Geometry: final body of the model. Coordinates: model frame, mm. A direction names the side the tool comes from. Give positions to 0.01 mm unless a question says otherwise; leave off trailing zeros. Write each loop counter-clockwise with the first axis right and the second up, starting at its lowest first coordinate (ties: lowest second). Pieces come first, ordered by that corner, then holes.
from build123d import *

# Parameters (mm, degrees)
SKETCH1_W                                           = 175
SKETCH1_H                                           = 77
BOSS_EXTRUDE1_DEPTH                                 = 10
CBORE_FOR_M5_HEX_SOCKET_HEAD_CAP_SCREW3_D           = 5.5
CBORE_FOR_M5_HEX_SOCKET_HEAD_CAP_SCREW3_CBORE_D     = 10
CBORE_FOR_M5_HEX_SOCKET_HEAD_CAP_SCREW3_CBORE_DEPTH = 5.4
M4_CLEARANCE_HOLE1_D                                = 4.5
CUT_EXTRUDE1_DEPTH                                  = 3.5
M4_CLEARANCE_HOLE2_D                                = 4.5
CUT_EXTRUDE2_DEPTH                                  = 3.5


with BuildPart() as part:
    # Sketch1 → Boss-Extrude1 (new body)
    with BuildSketch(Plane(origin=(0, 0, 0), x_dir=(1, 0, 0), z_dir=(0, 1, 0))):
        Rectangle(SKETCH1_W, SKETCH1_H)
    extrude(amount=BOSS_EXTRUDE1_DEPTH)

    # CBORE for M5 Hex Socket Head Cap Screw3 (through all)
    with Locations(Plane(origin=(-81.75, 10, 7.5), x_dir=(0, 0, 1), z_dir=(0, 1, 0))):
        with Locations((0, 0), (-15, 0), (-15, 30.5), (0, 30.5), (0, 133), (-15, 133), (-15, 163.5), (0, 163.5)):
            CounterBoreHole(CBORE_FOR_M5_HEX_SOCKET_HEAD_CAP_SCREW3_D / 2, CBORE_FOR_M5_HEX_SOCKET_HEAD_CAP_SCREW3_CBORE_D / 2, CBORE_FOR_M5_HEX_SOCKET_HEAD_CAP_SCREW3_CBORE_DEPTH)

    # M4 Clearance Hole1 (through all)
    with Locations(Plane(origin=(77.5, 10, 31.75), x_dir=(0, 0, 1), z_dir=(0, 1, 0))):
        with Locations((0, 0), (-65.21, 0)):
            Hole(M4_CLEARANCE_HOLE1_D / 2)

    # Sketch9 → Cut-Extrude1 (cut)
    with BuildSketch(Plane.XZ):
        Polygon((81.830127019, 31.75), (79.665063509, 35.5), (75.334936491, 35.5), (73.169872981, 31.75), (75.334936491, 28), (79.665063509, 28), align=None)
        Polygon((79.665063509, -29.71), (75.334936491, -29.71), (73.169872981, -33.46), (75.334936491, -37.21), (79.665063509, -37.21), (81.830127019, -33.46), align=None)
    extrude(amount=-CUT_EXTRUDE1_DEPTH, mode=Mode.SUBTRACT)

    # M4 Clearance Hole2 (through all)
    with Locations(Plane(origin=(-27.5, 0, 19), x_dir=(0, 0, -1), z_dir=(0, -1, 0))):
        with Locations((0, 0), (0, 55), (38, 0), (38, 55)):
            Hole(M4_CLEARANCE_HOLE2_D / 2)

    # Sketch12 → Cut-Extrude2 (cut)
    with BuildSketch(Plane(origin=(0, 10, 0), x_dir=(1, 0, 0), z_dir=(0, 1, 0))):
        Polygon((-23.169872981, 19), (-25.334936491, 22.75), (-29.665063509, 22.75), (-31.830127019, 19), (-29.665063509, 15.25), (-25.334936491, 15.25), align=None)
        Polygon((31.830127019, 19), (29.665063509, 22.75), (25.334936491, 22.75), (23.169872981, 19), (25.334936491, 15.25), (29.665063509, 15.25), align=None)
        Polygon((31.830127019, -19), (29.665063509, -15.25), (25.334936491, -15.25), (23.169872981, -19), (25.334936491, -22.75), (29.665063509, -22.75), align=None)
        Polygon((-23.169872981, -19), (-25.334936491, -15.25), (-29.665063509, -15.25), (-31.830127019, -19), (-29.665063509, -22.75), (-25.334936491, -22.75), align=None)
    extrude(amount=-CUT_EXTRUDE2_DEPTH, mode=Mode.SUBTRACT)


solid = part.part
Q1. Pin query (flat end, axial travel): P1, Ø4, axis at x = -28.5, z = 19, coming from the +Y side; P2, Ø8, axis at x = 51.5, z = -7, coming from the +Y side; P3, Ø4, axis at x = 77.5, z = 30.5, coming from the -Y side. Return the tip coordinate at first contact, or that it passes through.
Filled sheet:
P1: stops at y = 6.5
P2: stops at y = 4.6
P3: stops at y = 3.5
Q2. Access query for faces 4 (the flat face through (78, 2, 35.5)), 5 (the cylindrical face through (-29.496, 3.296, 20.038)), 6 (the flat face through (-30.732, 8.274, 17.099)). Directions: +Z, -Z, +X, -X, +Y, -Y. A direction counts if a zero-diameter tool reaches every point of the face in a straight line with its end or side. Return the directions, or none.
Filled sheet:
face 4: -Y
face 5: +Y, -Y
face 6: +Y
Q3. Pull-direction query (X, two-part tool) for faces 1 (the flat face through (-87.5, 5, 1)), 2 (the flat face through (27, 8, 22.75)), 3 (the flat face through (-1, 10, -1)); classes: released by +X, released by -X, zero draft, split by the parting line, or undercut.
Filled sheet:
face 1: released by -X
face 2: undercut
face 3: zero draft
Q4. Section C-C on x = 27.5. Output: boundary loops of the cut face in (y, z).
Filled sheet:
outline: (0, -38.5) - (10, -38.5) - (10, -22.75) - (6.5, -22.75) - (6.5, -21.25) - (0, -21.25) - close; (0, -16.75) - (6.5, -16.75) - (6.5, -15.25) - (10, -15.25) - (10, 15.25) - (6.5, 15.25) - (6.5, 16.75) - (0, 16.75) - close; (0, 21.25) - (6.5, 21.25) - (6.5, 22.75) - (10, 22.75) - (10, 38.5) - (0, 38.5) - close
Q5. Section A-A on x = 51.25. Output: boundary loops of the cut face in (y, z), plus the area to 3 significant figures.
Filled sheet:
outline: (0, -38.5) - (10, -38.5) - (10, -12.5) - (4.6, -12.5) - (4.6, -10.25) - (0, -10.25) - close; (0, -4.75) - (4.6, -4.75) - (4.6, -2.5) - (10, -2.5) - (10, 2.5) - (4.6, 2.5) - (4.6, 4.75) - (0, 4.75) - close; (0, 10.25) - (4.6, 10.25) - (4.6, 12.5) - (10, 12.5) - (10, 38.5) - (0, 38.5) - close
area: 611 mm2
Q6. Section B-B on z = 7.5. Count the separate pieces of the cut face and the enclosed holes in it, plus the area to 3 significant figures.
Filled sheet:
separate pieces: 5
enclosed holes: 0
area: 1,430 mm2
Q7. Ray query, line 1 along X through (y, z) = (6.4, -7.5); line 2 along X through (y, z) = (1, 7.5); line 3 along X through (y, z) = (7.25, -17.5). Return the intervals inside material, ascending.
Filled sheet:
line 1: x = -87.5 to -86.75, -76.75 to -56.25, -46.25 to 46.25, 56.25 to 76.75, 86.75 to 87.5
line 2: x = -87.5 to -84.5, -79 to -54, -48.5 to 48.5, 54 to 79, 84.5 to 87.5
line 3: x = -87.5 to -30.96, -24.04 to 24.04, 30.96 to 87.5
